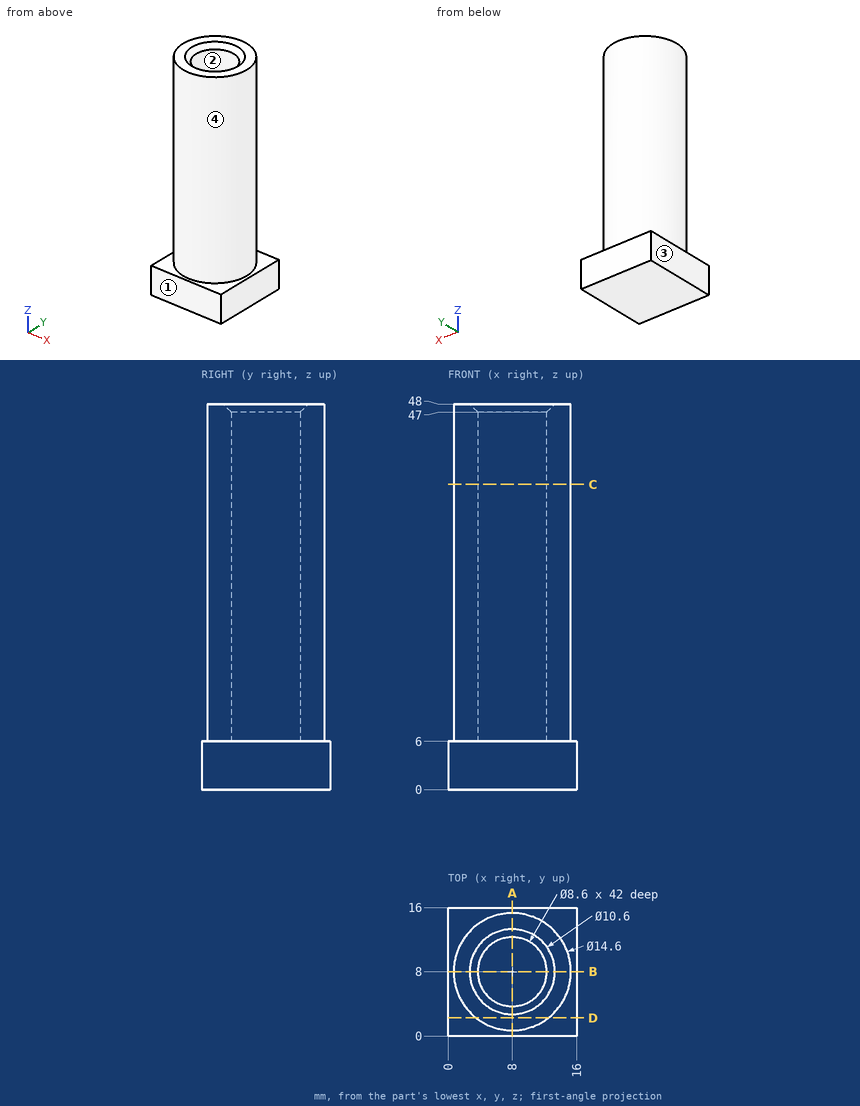
Design review of the part shown in the three views and the two pictorial views. Dimensions are in mm from the part's minimum x, y and z. Give positions to 0.01 mm unless a question says otherwise; leave off trailing zeros. Loops run counter-clockwise (first coordinate to the right, second up) from the corner with the lowest first, then second, coordinate; pieces in that order, holes last. Notation, with made-up numbers: (-22, -12) -> (22, -12) arc R8 ccw to (22, -3) -> close; hole circle Ø6 at (15.25, -5.75). An arc over 180 degrees is marked (long way). Put each result on its own line as item: value. Start each with the question number.
1. We need section D-D on y = 2.25. State the section outline as (x, z) points.
2. Wall thickness on probe 1 along Y at (x, z) = (8, 37); probe 2 along X at (y, z) = (9.75, 19); probe 3 along Z at (x, y) = (7, 5.25): over which ranges is each line inside the solid? List them lowest first.
3. We need section C-C on z = 38. State the section outline as (x, y) points.
4. Mouldability with a two-part tool opening along Y and no side actions: class the marked faces 1, 2, 3 and 4 as released by +Y, released by -Y, zero draft, split by the parting line, or undercut.
5. We need section A-A on x = 8. State the section outline as (y, z) points.
6. Clearance check with flat-ended pins moving along their axes: P1, Ø5, axis at y = 9, z = 27, coming from the +X side; P2, Ø7, axis at x = 8, y = 8, coming from the -Z side; P3, Ø5, axis at y = 12, z = 28.5, coming from the -X side; P4, Ø4, axis at y = 3.5, z = 40.5, coming from the -X side. State where each tip first meets the part, or that it passes through.
Determined:
1. outline: (0, 0) -> (16, 0) -> (16, 6) -> (12.5, 6) -> (12.5, 48) -> (3.5, 48) -> (3.5, 6) -> (0, 6) -> close
2. probe 1: 0.7 to 3.7, 12.3 to 15.3
2. probe 2: 0.91 to 4.07, 11.93 to 15.09
2. probe 3: 0 to 6
3. outline: circle Ø14.6 at (8, 8); hole circle Ø8.6 at (8, 8)
4. face 1: released by -Y
4. face 2: undercut
4. face 3: zero draft
4. face 4: split by the parting line
5. outline: (0, 0) -> (16, 0) -> (16, 6) -> (15.3, 6) -> (15.3, 48) -> (13.3, 48) -> (12.3, 47) -> (12.3, 6) -> (3.7, 6) -> (3.7, 47) -> (2.7, 48) -> (0.7, 48) -> (0.7, 6) -> (0, 6) -> close
6. P1: x = 15.3
6. P2: z = 0
6. P3: x = 0.86
6. P4: x = 1.14
